The listing builds one solid part. Answer for the finished solid, in the listing's coordinates (mm). Coordinates: 2 decimals unless noted, no trailing zeros. Write each loop counter-clockwise with the first axis right and the second up, starting at its lowest first coordinate (ties: lowest second). Pieces come first, ordered by that corner, then holes.
```python
from build123d import *

# Parameters (mm, degrees)
F0_R     = 26.5
F1_DEPTH = 20
F2_R     = 4
F3_DEPTH = 26.501
F4_DEPTH = 26.501


with BuildPart() as f1:
    # F0 (on Front) → F1 (new body)
    with BuildSketch(Plane.XZ):
        Circle(F0_R)
    extrude(amount=F1_DEPTH)

    # F2 (on Top) → F3 (cut, through all)
    with BuildSketch(Plane.XY):
        with Locations((0, -10)):
            Circle(F2_R)
    extrude(amount=-F3_DEPTH, mode=Mode.SUBTRACT)

    # F2 (on Top) → F4 (cut, through all)
    with BuildSketch(Plane.XY):
        with Locations((0, -10)):
            Circle(F2_R)
    extrude(amount=F4_DEPTH, mode=Mode.SUBTRACT)


solid = f1.part
```
(1) Find the intervals of material crossed by probe 1 along Y at (x, z) = (0, 8); probe 2 along X at (y, z) = (-10, -12.5); probe 3 along X at (y, z) = (-7, -6), in increasing order.
(2) Section A-A, the plane x = 0 is taken. Write down the section's boundary in (y, z), plus the area to 3 significant figures.
(3) Section C-C, the plane y = -1.5 is taken. Write down the section's boundary in (x, z), plus the area to 3 significant figures.
(4) Each of these flat-tipped pins is pushed along its axis until it touches: pin 1 (12 mm diameter, centred on y = -10.5, z = 17, fed in from +X); pin 2 (12 mm diameter, centred on x = 8.5, y = -3.5, fed in from -Z); pin 3 (5 mm diameter, centred on y = -5.5, z = -1, fed in from -X); pin 4 (2 mm diameter, centred on x = -6, y = -16, fed in from -Z). Where does it stop, or does it pass through?
(5) Section B-B, the plane z = 5 is taken. Write down the section's boundary in (x, y), plus the area to 3 significant figures.
(6) Section D-D, the plane y = -8.75 is taken. Write down the section's boundary in (x, z), plus the area to 3 significant figures.
Solution:
1. probe 1: y = -20 to -14, -6 to 0
1. probe 2: x = -23.37 to -4, 4 to 23.37
1. probe 3: x = -25.81 to -2.65, 2.65 to 25.81
2. outline: (-20, -26.5) - (-14, -26.5) - (-14, 26.5) - (-20, 26.5) - close; (-6, -26.5) - (0, -26.5) - (0, 26.5) - (-6, 26.5) - close
2. area: 636 mm2
3. outline: circle Ø53 at (0, 0)
3. area: 2,210 mm2
4. pin 1: stops at x = 24.11
4. pin 2: stops at z = -26.38
4. pin 3: stops at x = -26.5
4. pin 4: stops at z = -26.02
5. outline: (-26.02, -20) - (26.02, -20) - (26.02, 0) - (-26.02, 0) - close; hole circle Ø8 at (0, -10)
5. area: 991 mm2
6. outline: (-3.8, -26.23) - (-3.8, 26.23) arc R26.5 ccw to start; (3.8, -26.23) arc R26.5 ccw to (3.8, 26.23) - close
6. area: 1,800 mm2
